CAD build for the part. Positions are in the model's coordinates, mm. A direction names the side the tool comes from. Round coordinates to 2 decimals unless told otherwise and drop trailing zeros. Loops run counter-clockwise (first coordinate to the right, second up) from the corner with the lowest first, then second, coordinate; pieces in that order, holes last.
from build123d import *

# Parameters (mm, degrees)
BOSS_EXTRUDE1_DEPTH = 35
SKETCH2_R           = 1.75
CUT_EXTRUDE1_DEPTH  = 10
MOUNTING_WING_DEPTH = 2
SKETCH5_R           = 1.75
CUT_EXTRUDE2_DEPTH  = 3.5


with BuildPart() as part:
    # Sketch1 → Boss-Extrude1 (new body)
    with BuildSketch(Plane(origin=(0, 0, 0), x_dir=(1, 0, 0), z_dir=(0, 1, 0))):
        Polygon((-11.683800623, 0), (11.683800623, 0), (11.683800623, 14.5), (8.683800623, 14.5), (7.5, 12.3), (7.5, 9.3), (10, 9.3), (10, 1.5), (-10, 1.5), (-10, 9.3), (-7.5, 9.3), (-7.5, 12.3), (-8.683800623, 14.5), (-11.683800623, 14.5), align=None)
    extrude(amount=BOSS_EXTRUDE1_DEPTH)

    # Sketch2 → Cut-Extrude1 (cut)
    with BuildSketch(Plane.XY):
        with Locations((0, 5)):
            Circle(SKETCH2_R)
        with Locations((0, 24)):
            Circle(SKETCH2_R)
        with Locations((0, 11)):
            Circle(SKETCH2_R)
        with Locations((0, 30)):
            Circle(SKETCH2_R)
    extrude(amount=-CUT_EXTRUDE1_DEPTH, mode=Mode.SUBTRACT)

    # Optical Mount → Mounting Wing (add)
    with BuildSketch(Plane.ZY.offset(11.683800623)):
        Polygon((0, 0), (10, 0), (10, 35), (0, 35), (-14.5, 35), (-14.5, 0), align=None)
    extrude(amount=MOUNTING_WING_DEPTH)

    # Sketch5 → Cut-Extrude2 (cut)
    with BuildSketch(Plane(origin=(-11.683800623, 0, 0), x_dir=(0, 0, -1), z_dir=(1, 0, 0))):
        with Locations((-5, 4.5)):
            Circle(SKETCH5_R)
        with Locations((-5, 11.5)):
            Circle(SKETCH5_R)
        with Locations((-5, 23.5)):
            Circle(SKETCH5_R)
        with Locations((-5, 30.5)):
            Circle(SKETCH5_R)
    extrude(amount=-CUT_EXTRUDE2_DEPTH, mode=Mode.SUBTRACT)


solid = part.part
Item 1: Cut at B-B (z = 5). List the corners of the cut face in (x, y).
Verdict:
outline: (-13.68, 0) - (-11.68, 0) - (-11.68, 2.75) - (-13.68, 2.75) - close; (-13.68, 6.25) - (-11.68, 6.25) - (-11.68, 9.75) - (-13.68, 9.75) - close; (-13.68, 13.25) - (-11.68, 13.25) - (-11.68, 21.75) - (-13.68, 21.75) - close; (-13.68, 25.25) - (-11.68, 25.25) - (-11.68, 28.75) - (-13.68, 28.75) - close; (-13.68, 32.25) - (-11.68, 32.25) - (-11.68, 35) - (-13.68, 35) - close
Item 2: Cut at D-D (y = 30). List the corners of the cut face in (x, z), plus the area to 3 significant figures.
Verdict:
outline: (-13.68, -14.5) - (-8.68, -14.5) - (-7.5, -12.3) - (-7.5, -9.3) - (-10, -9.3) - (-10, -1.5) - (-1.75, -1.5) - (-1.75, 0) - (-11.68, 0) - (-11.68, 3.32) - (-13.68, 3.32) - close; (-13.68, 6.68) - (-11.68, 6.68) - (-11.68, 10) - (-13.68, 10) - close; (1.75, -1.5) - (10, -1.5) - (10, -9.3) - (7.5, -9.3) - (7.5, -12.3) - (8.68, -14.5) - (11.68, -14.5) - (11.68, 0) - (1.75, 0) - close
area: 139 mm2
Item 3: Mould opens along Y. For faces 1 (the cylindrical face through (-12.67, 31.68, 6.29)), 2 (the flat face through (-3, 35, -1)), 3 (the flat face through (-7.5, 17, -11)), 4 (the cylindrical face through (-0.228, 12.735, -0.74)) say: released by +Y, released by -Y, zero draft, split by the parting line, or undercut.
Verdict:
face 1: undercut
face 2: released by +Y
face 3: zero draft
face 4: undercut
Item 4: Cut at C-C (z = -3.75). List the corners of the cut face in (x, y), plus the area to 3 significant figures.
Verdict:
outline: (-13.68, 0) - (-10, 0) - (-10, 35) - (-13.68, 35) - close; (10, 0) - (11.68, 0) - (11.68, 35) - (10, 35) - close
area: 188 mm2
Item 5: Cut at A-A (x = 0). List the corners of the cut face in (y, z), plus the area to 3 significant figures.
Verdict:
outline: (0, -1.5) - (3.25, -1.5) - (3.25, 0) - (0, 0) - close; (6.75, -1.5) - (9.25, -1.5) - (9.25, 0) - (6.75, 0) - close; (12.75, -1.5) - (22.25, -1.5) - (22.25, 0) - (12.75, 0) - close; (25.75, -1.5) - (28.25, -1.5) - (28.25, 0) - (25.75, 0) - close; (31.75, -1.5) - (35, -1.5) - (35, 0) - (31.75, 0) - close
area: 31.5 mm2
Item 6: Flat gauge pins, fed straight in: P1, Ø3, axis at y = 21, z = 5, coming from the +X side; P2, Ø4.5, axis at x = 0, y = 5, coming from the -Z side; P3, Ø2, axis at y = 4.5, z = 5, coming from the -X side (3 decimals); P4, Ø12, axis at x = 7, y = 12, coming from the +Z side. Where does each tip first touch, or does it go through?
Verdict:
P1: stops at x = -11.68
P2: stops at z = -1.5
P3: passes through
P4: stops at z = 0
Item 7: Wall check: L1, parallel to Y at x = -12.35, z = 5; L2, parallel to Y at x = 0, z = -0.65; L3, parallel to X at y = 10, z = -7. Give the ranges that are in metal, low to high.
Verdict:
L1: y = 0 to 2.75, 6.25 to 9.75, 13.25 to 21.75, 25.25 to 28.75, 32.25 to 35
L2: y = 0 to 3.25, 6.75 to 9.25, 12.75 to 22.25, 25.75 to 28.25, 31.75 to 35
L3: x = -13.68 to -10, 10 to 11.68
Item 8: 3-axis set-ups, long thin cutter, end or side, ignore diameter. For faces 5 (the flat face through (-11.684, 18, 5)), 6 (the flat face through (-10, 17, -5)), 7 (the flat face through (11.684, 17, -7)), 8 (the flat face through (-8.08, 17.26, -13.38)): which of +Z, -Z, +X, -X, +Y, -Y reach the whole face in a straight line?
Verdict:
face 5: +Z, +X, +Y, -Y
face 6: +Y, -Y
face 7: +Z, -Z, +X, +Y, -Y
face 8: -Z, +Y, -Y
